Part print with two shaded views. Sizes in mm from the minimum x, y, z corner. A direction names the side the tool comes from. Give positions to 0.01 mm unless a question says otherwise; leave off trailing zeros. Write each loop counter-clockwise with the first axis right and the second up, starting at its lowest first coordinate (ties: lowest second). Pieces come first, ordered by that corner, then holes. Notation, with made-up numbers: M 28,67 L 74,67 A20 ccw 74,86 Z; hole C 68,55 d6. An arc over 180 degrees is marked long. Return JSON: item names as keys, results as strings. Group by question number.
Q1. Band-saw the part on C-C, the plane x = 90.5. Give the cut face in (y, z) (1 decimal).
Q2. Band-saw the part on B-B, the plane y = 95. Give the cut face in (x, z), then the cut area to 3 significant figures.
Q3. Tool access for the marked faces 1 and 2: list every direction of +Z, -Z, +X, -X, +Y, -Y with a clear straight run to the whole face (end or side of a thin tool).
Q4. Wall check: probe 1 along Z at (x, y) = (76, 143.5); probe 2 along Y at (x, z) = (85, 55); probe 3 along Y at (x, z) = (109.5, 26.5). Give the ranges that are in metal, low to high.
Q5. Flat gauge pins, fed straight in: pin 1 Ø10 at (x, z) = (104, 16.5) entering from +Y; pin 2 Ø8 at (y, z) = (59.5, 25.5) entering from +X; pin 3 Ø5 at (x, y) = (114.5, 36.5) entering from +Z. Where does each tip first touch, or does it go through?
Q6. Band-saw the part on D-D, the plane z = 6. Give the cut face in (x, y), then the cut area to 3 significant figures.
Q7. Pull direction X, two halves, no side cores. Call the marked faces 3, 4 and 5: +X half, -X half, draft (parallel to the pull), parting line (faces both ways), or undercut.
Q8. Band-saw the part on A-A, the plane z = 27.5. Give the cut face in (x, y).
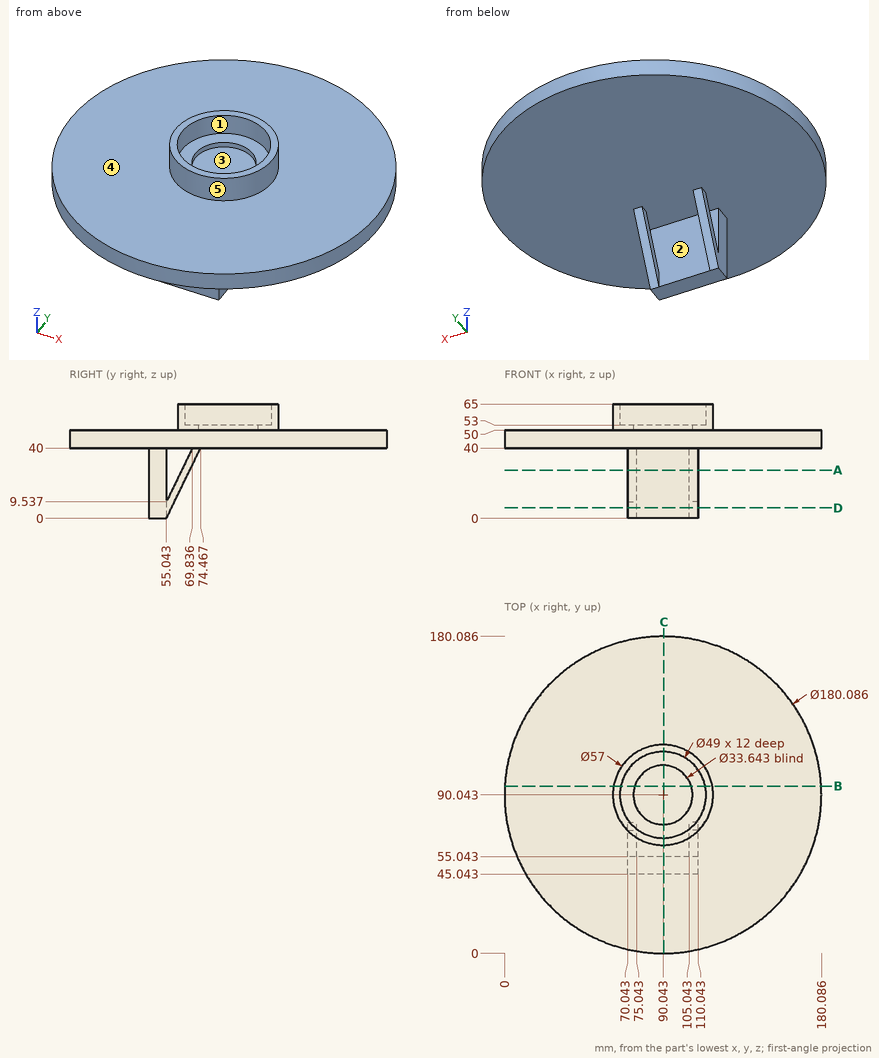
From the geometry:
{
 "1": {"outline": "M 0,40 L 45,40 L 45,0 L 55,0 L 55,40 L 180.1,40 L 180.1,50 L 118.5,50 L 118.5,65 L 114.5,65 L 114.5,53 L 106.9,53 L 106.9,50 L 73.2,50 L 73.2,53 L 65.5,53 L 65.5,65 L 61.5,65 L 61.5,50 L 0,50 Z"},
 "2": {"outline": "M 0.14,40 L 179.95,40 L 179.95,50 L 118.11,50 L 118.11,65 L 114.04,65 L 114.04,53 L 106.12,53 L 106.12,50 L 73.97,50 L 73.97,53 L 66.05,53 L 66.05,65 L 61.98,65 L 61.98,50 L 0.14,50 Z", "area": "1,970 mm^2"},
 "3": {"face 1": "+Z", "face 2": "none"},
 "4": {"probe 1": "z = 40 to 50", "probe 2": "y = 61.99 to 66.07, 114.02 to 118.09", "probe 3": "y = 45.04 to 55.04, 63.28 to 67.91"},
 "5": {"pin 1": "stops at y = 65.43", "pin 2": "stops at x = 110.04", "pin 3": "stops at z = 50"},
 "6": {"outline": "M 70.04,45.04 L 110.04,45.04 L 110.04,57.96 L 105.04,57.96 L 105.04,55.04 L 75.04,55.04 L 75.04,57.96 L 70.04,57.96 Z", "area": "429 mm^2"},
 "7": {"face 3": "undercut", "face 4": "draft", "face 5": "parting line"},
 "8": {"outline": "M 70.04,45.04 L 110.04,45.04 L 110.04,55.04 L 70.04,55.04 Z; M 70.04,63.77 L 75.04,63.77 L 75.04,68.4 L 70.04,68.4 Z; M 105.04,63.77 L 110.04,63.77 L 110.04,68.4 L 105.04,68.4 Z"}
}
